```python
from build123d import *

# Parameters (mm, degrees)
SKETCH1_W           = 8.55
SKETCH1_H           = 8.55
BOSS_EXTRUDE1_DEPTH = 8.3
SKETCH2_W           = 1.55
SKETCH2_H           = 1.4
CUT_EXTRUDE1_DEPTH  = 9.3
SKETCH3_W           = 1.3
SKETCH3_H           = 1.4
CUT_EXTRUDE2_DEPTH  = 9.55
SKETCH4_W           = 5.8
SKETCH4_H           = 5.8
CUT_EXTRUDE3_DEPTH  = 1.4
FILLET1_R           = 1.5
FILLET2_R           = 3
SKETCH5_R           = 1.75
CUT_EXTRUDE4_DEPTH  = 9.55
CHAMFER1_SIZE       = 0.5
CHAMFER1_SIZE2      = 0.350103769


with BuildPart() as part:
    # Sketch1 → Boss-Extrude1 (new body)
    with BuildSketch(Plane.XY):
        with Locations((4.275, 4.275)):
            Rectangle(SKETCH1_W, SKETCH1_H)
    extrude(amount=BOSS_EXTRUDE1_DEPTH)

    # Sketch2 → Cut-Extrude1 (cut, through all)
    with BuildSketch(Plane.XY.offset(8.3)):
        with Locations((0.775, 7.85)):
            Rectangle(SKETCH2_W, SKETCH2_H)
    extrude(amount=-CUT_EXTRUDE1_DEPTH, mode=Mode.SUBTRACT)

    # Sketch3 → Cut-Extrude2 (cut, through all)
    with BuildSketch(Plane(origin=(8.55, 0, 0), x_dir=(0, 0, -1), z_dir=(1, 0, 0))):
        with Locations((-0.65, 7.85)):
            Rectangle(SKETCH3_W, SKETCH3_H)
    extrude(amount=-CUT_EXTRUDE2_DEPTH, mode=Mode.SUBTRACT)

    # Sketch4 → Cut-Extrude3 (cut)
    with BuildSketch(Plane(origin=(0, 8.55, 0), x_dir=(1, 0, 0), z_dir=(0, 1, 0))):
        with Locations((4.45, -4.2)):
            Rectangle(SKETCH4_W, SKETCH4_H)
    extrude(amount=-CUT_EXTRUDE3_DEPTH, mode=Mode.SUBTRACT)

    # Fillet1
    fillet1_edges = [part.edges().sort_by_distance(p)[0] for p in [
        (7.35, 7.85, 7.1),
    ]]
    fillet(fillet1_edges, radius=FILLET1_R)

    # Fillet2
    fillet2_edges = [part.edges().sort_by_distance(p)[0] for p in [
        (8.55, 4.275, 8.3),
    ]]
    fillet(fillet2_edges, radius=FILLET2_R)

    # Sketch5 → Cut-Extrude4 (cut, through all)
    with BuildSketch(Plane.XZ):
        with Locations((3.65, 3.65)):
            Circle(SKETCH5_R)
    extrude(amount=-CUT_EXTRUDE4_DEPTH, mode=Mode.SUBTRACT)

    # Chamfer1
    chamfer1_edges = [part.edges().sort_by_distance(p)[0] for p in [
        (1.9, 0, 3.65),
    ]]
    chamfer1_side = [part.faces().sort_by_distance(p)[0] for p in [
        (8.430839394, 0, 2.65),
    ]]
    chamfer(chamfer1_edges, length=CHAMFER1_SIZE, length2=CHAMFER1_SIZE2, reference=chamfer1_side[0])


solid = part.part
```
Source: CAD feature listing. Evaluate the final solid. Frame: model axes, mm. A direction names the side the tool comes from. Round coordinates to 2 decimals unless told otherwise and drop trailing zeros. Loops run counter-clockwise (first coordinate to the right, second up) from the corner with the lowest first, then second, coordinate; pieces in that order, holes last.
(1) Section query A-A (z = 3.65). Output: boundary loops of the cut face in (x, y), and give its area (3 significant figures).
From the geometry:
outline: (0, 0) - (1.4, 0) - (1.9, 0.35) - (1.9, 7.15) - (0, 7.15) - close; (5.4, 0.35) - (5.9, 0) - (8.55, 0) - (8.55, 8.55) - (7.35, 8.55) - (7.35, 7.15) - (5.4, 7.15) - close
area: 37.6 mm2
(2) Section query C-C (y = 4). Output: boundary loops of the cut face in (x, z).
From the geometry:
outline: (0, 0) - (8.55, 0) - (8.55, 5.3) arc R3 ccw to (5.55, 8.3) - (0, 8.3) - close; hole circle Ø3.5 at (3.65, 3.65)
(3) Section query B-B (x = 3.65). Output: boundary loops of the cut face in (y, z).
From the geometry:
outline: (0, 0) - (7.15, 0) - (7.15, 1.9) - (0.35, 1.9) - (0, 1.4) - close; (0, 5.9) - (0.35, 5.4) - (7.15, 5.4) - (7.15, 7.1) - (8.55, 7.1) - (8.55, 8.3) - (0, 8.3) - close
(4) Section query D-D (z = 6.5). Output: boundary loops of the cut face in (x, y).
From the geometry:
outline: (0, 0) - (8.3, 0) - (8.3, 8.55) - (7.05, 8.55) - (7.05, 7.15) - (0, 7.15) - close
(5) Contact query for flat-ended pins moving along their axis: pin 1 Ø1.1 at (x, y) = (3.5, 8) entering from -Z; pin 2 Ø0.6 at (x, y) = (8, 7.5) entering from -Z; pin 3 Ø1 at (x, z) = (5.5, 3) entering from +Y. Output: stop coordinate, or through.
From the geometry:
pin 1: stops at z = 7.1
pin 2: stops at z = 1.3
pin 3: stops at y = 7.15
(6) Material intervals for probe 1 along Z at (x, y) = (3.65, 5.75); probe 2 along X at (y, z) = (6, 6.5); probe 3 along Y at (x, z) = (1, 5.75), sorted ascending.
From the geometry:
probe 1: z = 0 to 1.9, 5.4 to 8.3
probe 2: x = 0 to 8.3
probe 3: y = 0 to 7.15
(7) Pull-direction query (X, two-part tool) for faces 1 (the cylindrical face through (5.267, 3.702, 2.98)), 2 (the flat face through (8.55, 4, 3)), 3 (the flat face through (6.1, 0, 4.1)); classes: +X half, -X half, draft (parallel to the pull), parting line (faces both ways), or undercut.
From the geometry:
face 1: undercut
face 2: +X half
face 3: draft
(8) Access query for faces 4 (the cylindrical face through (6.9, 7.84, 6.67)), 5 (the flat face through (8, 8, 1.3)), 6 (the flat face through (1.55, 8, 8)). Directions: +Z, -Z, +X, -X, +Y, -Y. A direction counts if a zero-diameter tool reaches every point of the face in a straight line with its end or side. Return the directions, or none.
From the geometry:
face 4: -Z, -X, +Y
face 5: -Z, +X, -X, +Y
face 6: +Z, -Z, -X, +Y
